Verification items for the finished model (mm, model axes). A direction names the side the tool comes from. Give positions to 0.01 mm unless a question says otherwise; leave off trailing zeros. Loops run counter-clockwise (first coordinate to the right, second up) from the corner with the lowest first, then second, coordinate; pieces in that order, holes last. Notation, with made-up numbers: (-23, 15) -> (15, 15) arc R24 ccw to (15, 44) -> close; hole circle Ø4 at (29.5, 6). An arc over 180 degrees is marked (long way). Answer in a Markdown table with one row per item. Add a question column.
Q1. Section check C-C on z = 1. Enter the section's corners in (x, y).
Q2. Set-up check for faces 1 (the face through (0, 0, 11)), 2 (the face through (-2, 2, 6)): record each of +Z, -Z, +X, -X, +Y, -Y from which the full face is reachable in a straight line by a thin tool's end or side.
Q3. Section check D-D on z = 8.5. Enter the section's corners in (x, y), and give its area (3 significant figures).
Q4. Gauge pin test, flat ends, axial feed: P1, Ø1, axis at y = -2.5, z = 10, coming from the +X side; P2, Ø1.5, axis at x = -1.5, y = 2, coming from the -Z side. Record the tip position at first contact, or that the pin passes through.
Q5. Material ranges on probe 1 along Y at (x, z) = (0, 3.75); probe 2 along X at (y, z) = (1.1, 8.5); probe 3 along Y at (x, z) = (-0.55, 6.5), recorded low to high.
```python
from build123d import *

# Parameters (mm, degrees)
F2_SIZE = 0.5


with BuildPart() as f1:
    # F0 (on Front) → F1 (revolve)
    with BuildSketch(Plane.XZ):
        Polygon((0, 0), (1.95, 0), (1.95, 6), (3, 6), (3, 11), (0, 11), align=None)
    revolve(axis=Axis((0, 0, 5.355328), (0, 0, -1)))

    # F2
    f2_edges = [f1.edges().sort_by_distance(p)[0] for p in [
        (-3, 0, 11),
        (-1.95, 0, 0),
    ]]
    chamfer(f2_edges, length=F2_SIZE)

    # F3 (on Front) → F4 (revolve, cut)
    with BuildSketch(Plane.XZ):
        Polygon((1.950481, 6), (2.505797, 6), (1.950481, 6.137104), align=None)
    revolve(axis=Axis((0, 0, 5.414517), (0, 0, -1)), mode=Mode.SUBTRACT)


solid = f1.part
```
Taken from the geometry:
| question | item | result |
|---|---|---|
| 1 | outline | circle Ø3.9 at (0, 0) |
| 2 | face 1 | +Z, +X, -X, +Y, -Y |
| 2 | face 2 | -Z |
| 3 | outline | circle Ø6 at (0, 0) |
| 3 | area | 28.3 mm² |
| 4 | P1 | stops at x = 2.24 |
| 4 | P2 | stops at z = 0.3 |
| 5 | probe 1 | y = -1.95 to 1.95 |
| 5 | probe 2 | x = -2.79 to 2.79 |
| 5 | probe 3 | y = -2.95 to 2.95 |
